Here's the drawing with two shaded views (mm, measured from the low corner). I have some questions. A direction names the side the tool comes from. Round coordinates to 2 decimals unless told otherwise and drop trailing zeros. Loops run counter-clockwise (first coordinate to the right, second up) from the corner with the lowest first, then second, coordinate; pieces in that order, holes last. Notation, with made-up numbers: (-4, 85.25) - (9, 85.25) arc R18 ccw to (9, 103.25) - close; hole circle Ø3 at (15, -23.5). An arc over 180 degrees is marked (long way). Use one line per item in the form item = value.
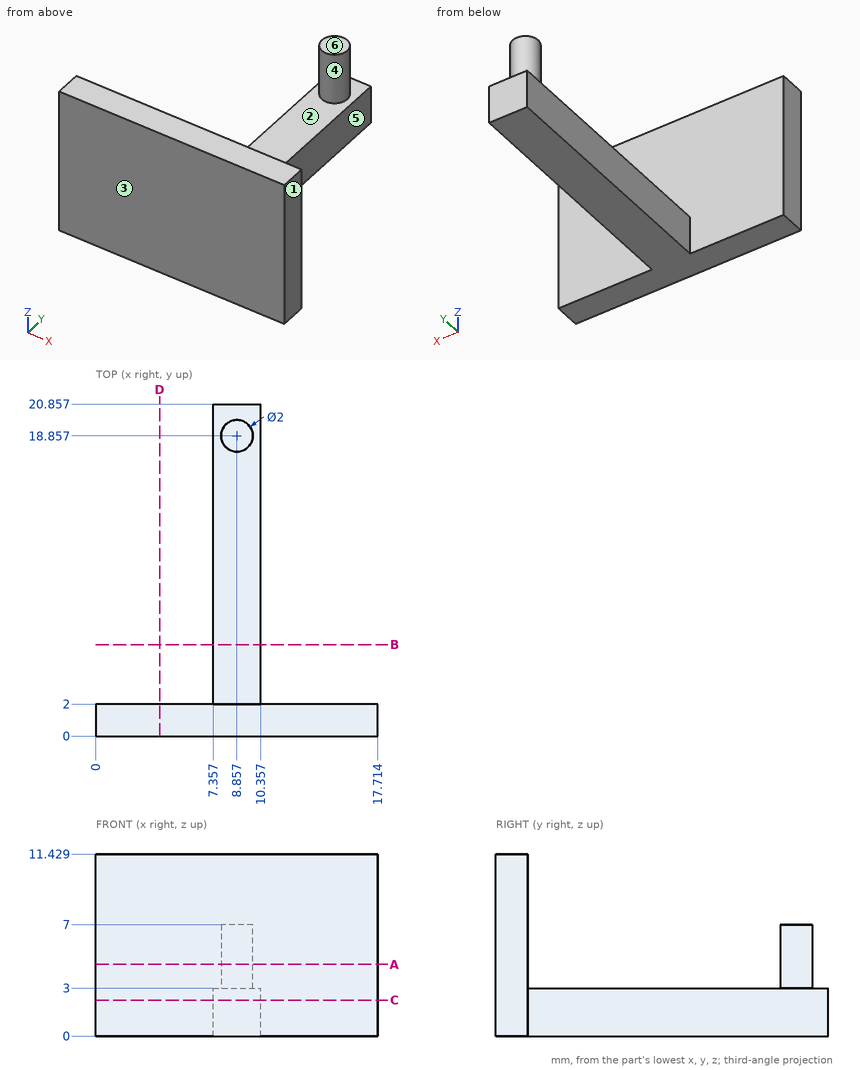
1. For P1, Ø2, axis at x = 11, z = 7, coming from the +Y side; P2, Ø0.9, axis at x = 9, y = 15.5, coming from the +Z side; P3, Ø4, axis at x = 6, z = 3, coming from the +Y side; P4, Ø0.9, axis at y = 13.5, z = 1.5, coming from the -X side, each with a flat end and sliding along its axis, tell me the tip position at first contact or that it passes through.
Solution:
P1 = 2
P2 = 3
P3 = 20.86
P4 = 7.36
2. If we section it at B-B, the plane y = 5.75: Write out the boundary of the cut face in (x, z).
Solution:
outline = (7.36, 0) - (10.36, 0) - (10.36, 3) - (7.36, 3) - close
3. We'd pull the mould along Y, two halves only. Please class the marked faces 1, 2 and 3: +Y half, -Y half, draft (parallel to the pull), parting line (faces both ways), or undercut.
Solution:
face_1 = draft
face_2 = undercut
face_3 = -Y half
4. If we section it at C-C, the plane z = 2.25: Write out the boundary of the cut face in (x, y) (1 decimal).
Solution:
outline = (0, 0) - (17.7, 0) - (17.7, 2) - (10.4, 2) - (10.4, 20.9) - (7.4, 20.9) - (7.4, 2) - (0, 2) - close
5. On a 3-axis mill with a long thin cutter (end or side, diameter ignored), from which of +Z, -Z, +X, -X, +Y, -Y can I reach the whole of each face in a straight line? I mean the marked faces 4, 5 and 6. Say none if no direction works.
Solution:
face_4 = +Z
face_5 = +Z, -Z, +X, +Y
face_6 = +Z, +X, -X, +Y
6. Please list where these lines run through material, in increasing order: line 1 along Y through (x, z) = (8.75, 4); line 2 along Y through (x, z) = (6, 5); line 3 along Z through (x, y) = (10.25, 5.75).
Solution:
line_1 = 0 to 2, 17.86 to 19.85
line_2 = 0 to 2
line_3 = 0 to 3
7. If we section it at A-A, the plane z = 4.5: Write out the boundary of the cut face in (x, y) (1 decimal).
Solution:
outline = (0, 0) - (17.7, 0) - (17.7, 2) - (0, 2) - close; circle Ø2 at (8.9, 18.9)
8. If we section it at D-D, the plane x = 4: Write out the boundary of the cut face in (y, z).
Solution:
outline = (0, 0) - (2, 0) - (2, 11.43) - (0, 11.43) - close
